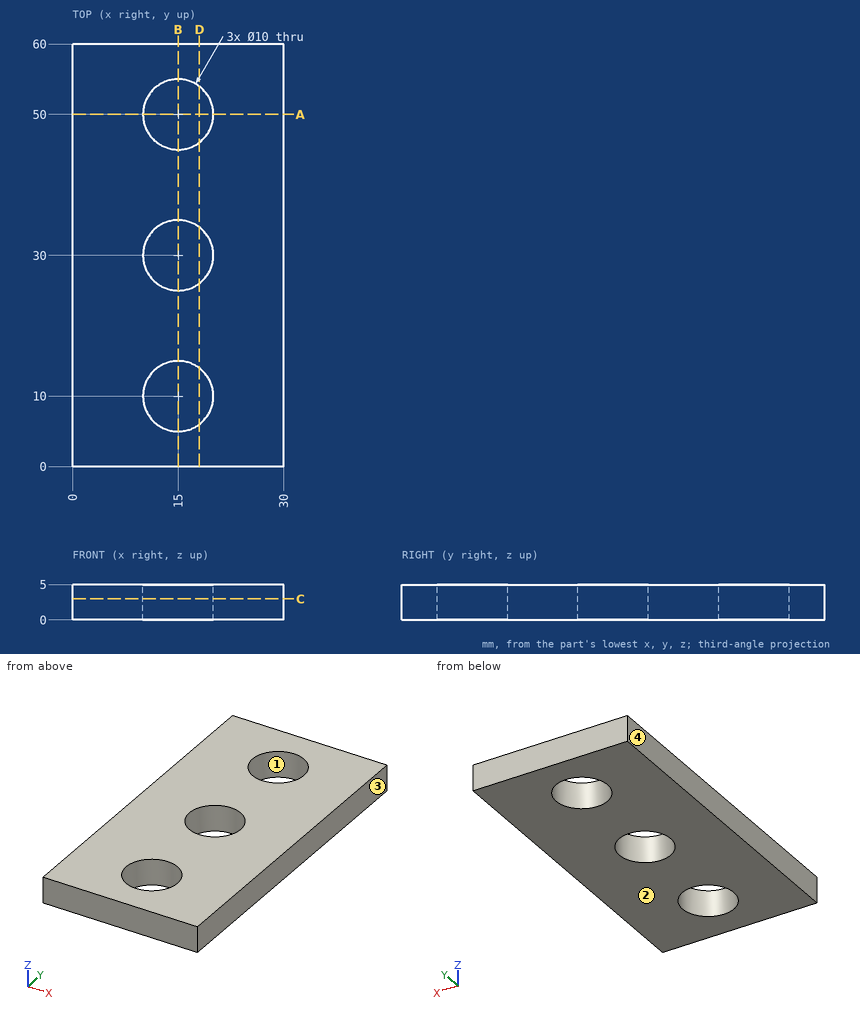
Geometry: see drawing. Coordinates: mm, zero at the bounding-box minimum. Give positions to 0.01 mm unless a question says otherwise; leave off trailing zeros. Loops run counter-clockwise (first coordinate to the right, second up) from the corner with the lowest first, then second, coordinate; pieces in that order, holes last. Notation, with made-up numbers: (80.5, 87) -> (127.5, 87) arc R10 ccw to (127.5, 93) -> close; hole circle Ø8 at (24.5, 62.25). An arc over 180 degrees is marked (long way). Answer as a JSON object with one key per item and string values. Group by question number.
Item 1: Pull-direction query (X, two-part tool) for the marked faces 1, 2, 3 and 4; classes: released by +X, released by -X, zero draft, split by the parting line, or undercut.
Item 2: Cut plane A-A, the plane y = 50. Return the cut outline in (x, z).
Item 3: Cut plane B-B, the plane x = 15. Return the cut outline in (y, z).
Item 4: Cut plane D-D, the plane x = 18. Return the cut outline in (y, z), and give its area (3 significant figures).
Item 5: Line query: probe 1 along Y at (x, z) = (15, 1.7); probe 2 along X at (y, z) = (49, 0.95); probe 3 along X at (y, z) = (45.5, 4.75). Output: solid intervals per line, ascending.
Item 6: Pin query (flat end, axial travel): P1, Ø11.5, axis at x = 15, y = 10, coming from the -Z side. Return the tip coordinate at first contact, or that it passes through.
Item 7: Cut plane C-C, the plane z = 3. Return the cut outline in (x, y), and give its area (3 significant figures).
Checks:
{
 "1": {"face 1": "undercut", "face 2": "zero draft", "face 3": "released by +X", "face 4": "released by -X"},
 "2": {"outline": "(0, 0) -> (10, 0) -> (10, 5) -> (0, 5) -> close; (20, 0) -> (30, 0) -> (30, 5) -> (20, 5) -> close"},
 "3": {"outline": "(0, 0) -> (5, 0) -> (5, 5) -> (0, 5) -> close; (15, 0) -> (25, 0) -> (25, 5) -> (15, 5) -> close; (35, 0) -> (45, 0) -> (45, 5) -> (35, 5) -> close; (55, 0) -> (60, 0) -> (60, 5) -> (55, 5) -> close"},
 "4": {"outline": "(0, 0) -> (6, 0) -> (6, 5) -> (0, 5) -> close; (14, 0) -> (26, 0) -> (26, 5) -> (14, 5) -> close; (34, 0) -> (46, 0) -> (46, 5) -> (34, 5) -> close; (54, 0) -> (60, 0) -> (60, 5) -> (54, 5) -> close", "area": "180 mm²"},
 "5": {"probe 1": "y = 0 to 5, 15 to 25, 35 to 45, 55 to 60", "probe 2": "x = 0 to 10.1, 19.9 to 30", "probe 3": "x = 0 to 12.82, 17.18 to 30"},
 "6": {"P1": "stops at z = 0"},
 "7": {"outline": "(0, 0) -> (30, 0) -> (30, 60) -> (0, 60) -> close; hole circle Ø10 at (15, 10); hole circle Ø10 at (15, 30); hole circle Ø10 at (15, 50)", "area": "1,560 mm²"}
}
